```python
from build123d import *

# Parameters (mm, degrees)
SKETCH_1_W          = 10
SKETCH_1_H          = 15.5
EXTRUDE_1_DEPTH     = 10
SKETCH_2_W          = 10
SKETCH_2_H          = 10
EXTRUDE_2_DEPTH     = 5
SKETCH_3_R          = 1.5
CUT_EXTRUDE_1_DEPTH = 5
SKETCH_4_R          = 1.5
CUT_EXTRUDE_2_DEPTH = 10


with BuildPart() as part:
    # 草图1 → 凸台-拉伸1 (new body)
    with BuildSketch(Plane.XY):
        Rectangle(SKETCH_1_W, SKETCH_1_H)
    extrude(amount=EXTRUDE_1_DEPTH)

    # 草图2 → 凸台-拉伸2 (add)
    with BuildSketch(Plane(origin=(0, 7.75, 0), x_dir=(1, 0, 0), z_dir=(0, 1, 0))):
        with Locations((0, -15)):
            Rectangle(SKETCH_2_W, SKETCH_2_H)
        with Locations((0, 5)):
            Rectangle(SKETCH_2_W, SKETCH_2_H)
    extrude(amount=-EXTRUDE_2_DEPTH)

    # 草图3 → 切除-拉伸1 (cut)
    with BuildSketch(Plane.XZ.offset(-2.75)):
        with Locations(Location((0, -5, 0), (0, 0, 270))):
            Circle(SKETCH_3_R)
        with Locations(Location((0, 15, 0), (0, 0, 270))):
            Circle(SKETCH_3_R)
    extrude(amount=-CUT_EXTRUDE_1_DEPTH, mode=Mode.SUBTRACT)

    # 草图4 → 切除-拉伸2 (cut)
    with BuildSketch(Plane.XY.offset(10)):
        with Locations((-2.5, -5.25)):
            Circle(SKETCH_4_R)
        with Locations((2.5, -1.75)):
            Circle(SKETCH_4_R)
    extrude(amount=-CUT_EXTRUDE_2_DEPTH, mode=Mode.SUBTRACT)


solid = part.part
```
Part model, mm, in its own coordinate system. A direction names the side the tool comes from. Give positions to 0.01 mm unless a question says otherwise; leave off trailing zeros. Order: outer loops, then holes, each group sorted by start corner. A loop starts at its lowest first (then second) coordinate and runs counter-clockwise, first axis right, second up. Notation, with made-up numbers: M 58,70 L 111,70 A18 ccw 111,83 Z; hole C -14,39.5 d5. An arc over 180 degrees is marked long. Use a Markdown table: item, result. Add a question column.
(1) Saw through at B-B, the plane z = 15. Give the cut face in (x, y).
(2) 3-axis set-ups, long thin cutter, end or side, ignore diameter. For faces 1 (the face through (-1.2, 2.75, -6.2)), 2 (the face through (0, 5, -10)), 3 (the face through (0, -2, 10)): which of +Z, -Z, +X, -X, +Y, -Y reach the whole face in a straight line?
(3) Probe line 1 along X through (y, z) = (4.4, 15); line 2 along Z through (x, y) = (0.25, -6); line 3 along X through (y, z) = (-3, 8.75). List the from-to ranges inside material, lowest first. Write a range as [from, to].
(4) Saw through at C-C, the plane x = -2.5. Give the cut face in (y, z).
(5) Mould opens along X. For faces 4 (the face through (5, 2, 5)), 5 (the face through (-0.575, 5.215, -6.386)), 6 (the face through (-5, 2, 5)), 7 (the face through (-1.2, 2.75, 13.8)) say: +X half, -X half, draft (parallel to the pull), parting line (faces both ways), or undercut.
(6) Drop flat-ended pins along their axis: P1, Ø3, axis at x = 2, y = -3.5, coming from the +Z side; P2, Ø5, axis at x = 2.5, z = -3.5, coming from the -Y side; P3, Ø2.5, axis at x = 0, z = -5, coming from the +Y side; P4, Ø4, axis at y = 2.5, z = -4.5, coming from the +X side. Give the stop position or say it passes through.
(7) Saw through at D-D, the plane z = 3.25. Give the cut face in (x, y), and give its area (3 significant figures).
(8) Saw through at A-A, the plane y = -5.25. Give the cut face in (x, z).
Answer key:
| question | item | result |
|---|---|---|
| 1 | outline | M -5,2.75 L -1.5,2.75 L -1.5,7.75 L -5,7.75 Z; M 1.5,2.75 L 5,2.75 L 5,7.75 L 1.5,7.75 Z |
| 2 | face 1 | -Z, +X, -X, -Y |
| 2 | face 2 | -Z, +X, -X, +Y, -Y |
| 2 | face 3 | +Z, +X, -X, -Y |
| 3 | line 1 | [-5, -1.5], [1.5, 5] |
| 3 | line 2 | [0, 10] |
| 3 | line 3 | [-5, 1.67], [3.33, 5] |
| 4 | outline | M -7.75,0 L -6.75,0 L -6.75,10 L -7.75,10 Z; M -3.75,0 L 2.75,0 L 2.75,-10 L 7.75,-10 L 7.75,20 L 2.75,20 L 2.75,10 L -3.75,10 Z |
| 5 | face 4 | +X half |
| 5 | face 5 | undercut |
| 5 | face 6 | -X half |
| 5 | face 7 | draft |
| 6 | P1 | z = 10 |
| 6 | P2 | y = 2.75 |
| 6 | P3 | through |
| 6 | P4 | x = 5 |
| 7 | outline | M -5,-7.75 L 5,-7.75 L 5,7.75 L -5,7.75 Z; hole C -2.5,-5.25 d3; hole C 2.5,-1.75 d3 |
| 7 | area | 141 mm^2 |
| 8 | outline | M -5,0 L -4,0 L -4,10 L -5,10 Z; M -1,0 L 5,0 L 5,10 L -1,10 Z |
